```python
from build123d import *

# Parameters (mm, degrees)
EXTRUDE_3_DEPTH      = 20
SKETCH_8_W           = 14
SKETCH_8_H           = 24.2
CUT_EXTRUDE_5_DEPTH  = 24.2
CUT_EXTRUDE_6_DEPTH  = 43.067089274
CUT_EXTRUDE_7_DEPTH  = 43.067089274
EXTRUDE_4_DEPTH      = 2.7
EXTRUDE_4_DEPTH_BACK = 2.7
SKETCH_11_W          = 2
SKETCH_11_H          = 2


with BuildPart() as part:
    # 草图7 → 凸台-拉伸3 (new body)
    with BuildSketch(Plane.XY):
        Polygon((0, 0), (0, 28), (6.5, 28), (6.5, 21.5), (21.5, 6.5), (28, 6.5), (28, 0), align=None)
    extrude(amount=EXTRUDE_3_DEPTH)

    # 草图8 → 切除-拉伸5 (cut)
    with BuildSketch(Plane(origin=(28, 0, 0), x_dir=(0, 0, -1), z_dir=(1, 0, 0))):
        with Locations((-10, 15.9)):
            Rectangle(SKETCH_8_W, SKETCH_8_H)
    extrude(amount=-CUT_EXTRUDE_5_DEPTH, mode=Mode.SUBTRACT)

    # 草图9 → 切除-拉伸6 (cut, through all)
    with BuildSketch(Plane(origin=(3.8, 0, 0), x_dir=(0, 0, -1), z_dir=(1, 0, 0))):
        with BuildLine():
            Line((-6.75, 18), (-6.75, 12))
            ThreePointArc((-6.75, 12), (-10, 8.75), (-13.25, 12))
            Line((-13.25, 12), (-13.25, 18))
            ThreePointArc((-13.25, 18), (-10, 21.25), (-6.75, 18))
        make_face()
    extrude(amount=-CUT_EXTRUDE_6_DEPTH, mode=Mode.SUBTRACT)

    # 草图10 → 切除-拉伸7 (cut, through all)
    with BuildSketch(Plane(origin=(0, 3.8, 0), x_dir=(1, 0, 0), z_dir=(0, 1, 0))):
        with BuildLine():
            Line((12, -6.75), (18, -6.75))
            ThreePointArc((18, -6.75), (21.25, -10), (18, -13.25))
            Line((18, -13.25), (12, -13.25))
            ThreePointArc((12, -13.25), (8.75, -10), (12, -6.75))
        make_face()
    extrude(amount=-CUT_EXTRUDE_7_DEPTH, mode=Mode.SUBTRACT)

    # 草图11 → 凸台-拉伸4 (add, two sides: drawn at the far end of the back side and taken through both)
    with BuildSketch(Plane.XY.offset(10).offset(-EXTRUDE_4_DEPTH_BACK)):
        with Locations((4.5, -1)):
            Rectangle(SKETCH_11_W, SKETCH_11_H)
        with Locations((23.5, -1)):
            Rectangle(SKETCH_11_W, SKETCH_11_H)
        with Locations((-1, 23.5)):
            Rectangle(SKETCH_11_W, SKETCH_11_H)
        with Locations((-1, 4.5)):
            Rectangle(SKETCH_11_W, SKETCH_11_H)
    extrude(amount=EXTRUDE_4_DEPTH + EXTRUDE_4_DEPTH_BACK)


solid = part.part
```
Source: CAD feature listing. Evaluate the final solid. Frame: model axes, mm. A direction names the side the tool comes from. Give positions to 0.01 mm unless a question says otherwise; leave off trailing zeros. Loops run counter-clockwise (first coordinate to the right, second up) from the corner with the lowest first, then second, coordinate; pieces in that order, holes last. Notation, with made-up numbers: M 76.5,84 L 126.5,84 A36 ccw 126.5,121 Z; hole C 81.5,21.25 d1. An arc over 180 degrees is marked long. Put each result on its own line as item: value.
Q1. Pin query (flat end, axial travel): P1, Ø1.6, axis at x = -1.5, y = 24, coming from the +Z side; P2, Ø0.9, axis at x = 23.5, z = 2, coming from the +Y side; P3, Ø1, axis at y = -1, z = 10.5, coming from the -X side. Return the tip coordinate at first contact, or that it passes through.
Response values:
P1: stops at z = 12.7
P2: stops at y = 6.5
P3: stops at x = 3.5
Q2. Line query: probe 1 along Z at (x, y) = (12.25, 3.5); probe 2 along Z at (x, y) = (5.5, 16.25); probe 3 along Y at (x, z) = (0.5, 18). Output: solid intervals per line, ascending. Write a range as [from, to].
Response values:
probe 1: z = [0, 6.75], [13.25, 20]
probe 2: z = [0, 3], [17, 20]
probe 3: y = [0, 28]
Q3. Mould query, pull axis Z, two halves, no side actions, for faces 5 (the flat face through (3.8, 16, 15)), 6 (the flat face through (-1, 5, 12.7)), 7 (the flat face through (28, 3, 10)). Classes: released by +Z, released by -Z, zero draft, split by the parting line, or undercut.
Response values:
face 5: undercut
face 6: released by +Z
face 7: zero draft
Q4. Section A-A (z = 10). Count the separate pieces of the cut face and the enclosed holes in it, and give its area (3 significant figures).
Response values:
separate pieces: 3
enclosed holes: 0
area: 119 mm²
Q5. Section B-B (x = 1). Return the cut outline in (y, z).
Response values:
outline: M 0,0 L 28,0 L 28,20 L 0,20 Z; hole M 12,6.75 L 18,6.75 A3.25 ccw 18,13.25 L 12,13.25 A3.25 ccw Z
Q6. Section D-D (x = 20.75). Return the cut outline in (y, z), and give its area (3 significant figures).
Response values:
outline: M 0,0 L 7.25,0 L 7.25,3 L 3.8,3 L 3.8,8.27 L 0,8.27 Z; M 0,11.73 L 3.8,11.73 L 3.8,17 L 7.25,17 L 7.25,20 L 0,20 Z
area: 83.5 mm²
Q7. Reachability of faces 1 (the flat face through (23, -1, 7.3)), 2 (the flat face through (15, 2, 6.75)), 3 (the flat face through (5.5, -1, 10)), 4 (the cylindrical face through (1.93, 21.25, 10.07)) from +Z, -Z, +X, -X, +Y, -Y: full face, straight path, thin tool, end or side. Return the list, or none.
Response values:
face 1: -Z, +X, -X, -Y
face 2: +Y, -Y
face 3: +Z, -Z, -Y
face 4: +X, -X
